Verification items for the finished model (mm, model axes). A direction names the side the tool comes from. Give positions to 0.01 mm unless a question says otherwise; leave off trailing zeros. Write each loop counter-clockwise with the first axis right and the second up, starting at its lowest first coordinate (ties: lowest second). Pieces come first, ordered by that corner, then holes. Notation, with made-up numbers: (57, 83) -> (83, 83) arc R17 cw to (83, 91) -> close; hole circle Ø6 at (-32.5, 40). An arc over 180 degrees is marked (long way). Answer as CSV lines item,"result". Start each with the question number.
1) Mould release check, pull along X, two halves, no side actions. Record for faces 3 (the flat face through (-45.81, 26.69, -13.52)), 4 (the flat face through (-31, -15, -19.812)), 5 (the flat face through (-15.13, 26.45, -13.52)): released by +X, released by -X, zero draft, split by the parting line, or undercut.
2) Gauge pin test, flat ends, axial feed: pin 1 Ø5.5 at (x, y) = (-22.5, 13) entering from +Z; pin 2 Ø2 at (x, z) = (-35.5, -19.5) entering from +Y; pin 3 Ø3 at (x, z) = (-11, -8.5) entering from +Y. Record the tip position at first contact, or that the pin passes through.
3) Sectioned sample at B-B on z = -17. Record the cut outline in (x, y).
4) Material ranges on L1, parallel to X at y = -1.5, z = -3.5; L2, parallel to Z at x = -48, y = 0; L3, parallel to Y at x = -32, z = -8.75, recorded low to high.
5) Sectioned sample at D-D on y = -24.5. Record the cut outline in (x, z), and give its area (3 significant figures).
6) Sectioned sample at C-C on x = -23. Record the cut outline in (y, z) (3 decimals).
7) Sectioned sample at A-A on y = 0. Record the cut outline in (x, z).
8) Tool access check on faces 1 (the flat face through (-31, 0, -27.432)), 2 (the flat face through (-31, 15, -19.812)). Record the directions out of +Z, -Z, +X, -X, +Y, -Y that give a thin tool (end or side, any length) a straight path to the whole face; none if there is none.
```python
from build123d import *

# Parameters (mm, degrees)
F2_DEPTH = 27.432
F3_T     = -7.62
F4_D     = 19.05


with BuildPart() as f2:
    # F1 (on Top) → F2 (new body)
    with BuildSketch(Plane.XY):
        Polygon((0, -17.71341), (0, 17.71341), (-30.680526, 35.42682), (-61.361052, 17.71341), (-61.361052, -17.71341), (-30.680526, -35.42682), align=None)
    extrude(amount=-F2_DEPTH)

    # F3
    f3_openings = [f2.faces().sort_by_distance(p)[0] for p in [
        (-30.680526, 0, 0),
    ]]
    offset(amount=F3_T, openings=f3_openings)

    # F4 (through all)
    with Locations(Plane.YZ):
        with Locations((0, -14.139283)):
            Hole(F4_D / 2)


solid = f2.part
```
Ans:
1,face 3,"released by -X"
1,face 4,"undercut"
1,face 5,"released by +X"
2,pin 1,"stops at z = -19.81"
2,pin 2,"stops at y = 33.22"
2,pin 3,"stops at y = 24.93"
3,outline,"(-61.36, -17.71) -> (-30.68, -35.43) -> (0, -17.71) -> (0, -9.09) -> (-7.62, -9.09) -> (-7.62, -13.31) -> (-30.68, -26.63) -> (-53.74, -13.31) -> (-53.74, -9.09) -> (-61.36, -9.09) -> close; (-61.36, 9.09) -> (-53.74, 9.09) -> (-53.74, 13.31) -> (-30.68, 26.63) -> (-7.62, 13.31) -> (-7.62, 9.09) -> (0, 9.09) -> (0, 17.71) -> (-30.68, 35.43) -> (-61.36, 17.71) -> close"
4,L1,"x = -61.36 to -53.74, -7.62 to 0"
4,L2,"z = -27.43 to -23.66"
4,L3,"y = -34.67 to -25.87, 25.87 to 34.67"
5,outline,"(-49.61, -27.43) -> (-11.75, -27.43) -> (-11.75, 0) -> (-26.99, 0) -> (-26.99, -19.81) -> (-34.37, -19.81) -> (-34.37, 0) -> (-49.61, 0) -> close"
5,area,"892 mm²"
6,outline,"(-30.992, -27.432) -> (30.992, -27.432) -> (30.992, 0) -> (22.194, 0) -> (22.194, -19.812) -> (7.652, -19.812) arc R9.525 cw to (-7.652, -19.812) -> (-22.194, -19.812) -> (-22.194, 0) -> (-30.992, 0) -> close"
7,outline,"(-61.36, -27.43) -> (0, -27.43) -> (0, -23.66) -> (-61.36, -23.66) -> close; (-61.36, -4.61) -> (-53.74, -4.61) -> (-53.74, 0) -> (-61.36, 0) -> close; (-7.62, -4.61) -> (0, -4.61) -> (0, 0) -> (-7.62, 0) -> close"
8,face 1,"-Z, +X, -X, +Y, -Y"
8,face 2,"+Z"
